from build123d import *

# Parameters (mm, degrees)
SKETCH1_W           = 300
SKETCH1_H           = 200
BOSS_EXTRUDE1_DEPTH = 60
FILLET1_R           = 5
SHELL1_START        = -145
SHELL1_OUTLINE_W    = 190
SHELL1_OUTLINE_H    = 115
SHELL1_DEPTH        = 290
SKETCH5_W           = 110
SKETCH5_H           = 180
CUT_EXTRUDE1_DEPTH  = 2.5
SKETCH6_W           = 110
SKETCH6_H           = 180
CUT_EXTRUDE2_DEPTH  = 2.5
SKETCH7_R           = 8.25
CUT_EXTRUDE3_DEPTH  = 320.540685985


# Read off the part's stored shape, not the designer's step: Shell1
with BuildPart() as part:
    # Sketch1 → Boss-Extrude1 (new, symmetric)
    with BuildSketch(Plane.XY):
        Rectangle(SKETCH1_W, SKETCH1_H)
    extrude(amount=BOSS_EXTRUDE1_DEPTH, both=True)

    # Fillet1
    fillet1_edges = [part.edges().sort_by_distance(p)[0] for p in [
        (150, -100, 0),
        (-150, -100, 0),
        (-150, 100, 0),
        (150, 100, 0),
    ]]
    fillet(fillet1_edges, radius=FILLET1_R)

    # Shell1 outline → Shell1 (cut)
    with BuildSketch(Plane.YZ.offset(SHELL1_START)):
        with Locations((0, 2.5)):
            Rectangle(SHELL1_OUTLINE_W, SHELL1_OUTLINE_H)
    extrude(amount=SHELL1_DEPTH, mode=Mode.SUBTRACT)

    # Sketch5 → Cut-Extrude1 (cut)
    with BuildSketch(Plane(origin=(150, 0, 0), x_dir=(0, 0, -1), z_dir=(1, 0, 0))):
        Rectangle(SKETCH5_W, SKETCH5_H)
    extrude(amount=-CUT_EXTRUDE1_DEPTH, mode=Mode.SUBTRACT)

    # Sketch6 → Cut-Extrude2 (cut)
    with BuildSketch(Plane.ZY.offset(150)):
        Rectangle(SKETCH6_W, SKETCH6_H)
    extrude(amount=-CUT_EXTRUDE2_DEPTH, mode=Mode.SUBTRACT)

    # Sketch7 → Cut-Extrude3 (cut, through all)
    with BuildSketch(Plane.ZY.offset(147.5)):
        with Locations((0, 43.15529971)):
            Circle(SKETCH7_R)
        with Locations((0, -26.84470029)):
            Circle(SKETCH7_R)
    extrude(amount=-CUT_EXTRUDE3_DEPTH, mode=Mode.SUBTRACT)


solid = part.part
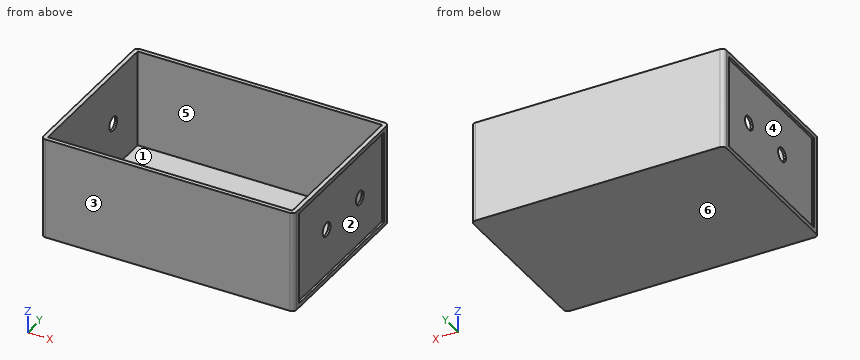
Could you check a few things on this model? Use its own coordinates, in mm. Face numbers are marked on the shaded views. A direction names the side the tool comes from. Coordinates: 2 decimals unless noted, no trailing zeros. Loops run counter-clockwise (first coordinate to the right, second up) from the corner with the lowest first, then second, coordinate; pieces in that order, holes last. Notation, with made-up numbers: (61, 9) -> (100, 9) arc R17 cw to (100, 39) -> close; hole circle Ø4 at (-29.75, -32.75). An arc over 180 degrees is marked (long way). Answer in a Markdown table with one row per item.
(1) For the marked faces 4, 5 and 6, which set-ups out of +Z, -Z, +X, -X, +Y, -Y let a thin tool reach every point of the face, with its end or its side?
Results found:
| item | result |
|---|---|
| face 4 | -X |
| face 5 | +Z |
| face 6 | -Z, +X, -X, +Y, -Y |
(2) Imagine slicing it at A-A (z = -49). List the corners of the cut face in (x, y) for me.
Results found:
| item | result |
|---|---|
| outline | (-150, -95) arc R5 ccw to (-145, -100) -> (145, -100) arc R5 ccw to (150, -95) -> (150, -90) -> (147.5, -90) -> (147.5, 90) -> (150, 90) -> (150, 95) arc R5 ccw to (145, 100) -> (-145, 100) arc R5 ccw to (-150, 95) -> (-150, 90) -> (-147.5, 90) -> (-147.5, -90) -> (-150, -90) -> close; hole (-145, -95) -> (145, -95) -> (145, 95) -> (-145, 95) -> close |
(3) Imagine slicing it at B-B (x = 99). List the corners of the cut face in (y, z) for me.
Results found:
| item | result |
|---|---|
| outline | (-100, -60) -> (100, -60) -> (100, 60) -> (95, 60) -> (95, -55) -> (-95, -55) -> (-95, 60) -> (-100, 60) -> close |
(4) Imagine slicing it at D-D (z = 0). Give the number of separate pieces and of enclosed holes in the cut face, plus the area to 3 significant figures.
Results found:
| item | result |
|---|---|
| separate pieces | 4 |
| enclosed holes | 0 |
| area | 3,810 mm^2 |
(5) Imagine slicing it at C-C (y = 71). List the corners of the cut face in (x, z) for me.
Results found:
| item | result |
|---|---|
| outline | (-150, -60) -> (150, -60) -> (150, -55) -> (147.5, -55) -> (147.5, 55) -> (150, 55) -> (150, 60) -> (145, 60) -> (145, -55) -> (-145, -55) -> (-145, 60) -> (-150, 60) -> (-150, 55) -> (-147.5, 55) -> (-147.5, -55) -> (-150, -55) -> close |
(6) If I drill on probe 1 along X at (y, z) = (8.5, -12.5); probe 2 along Y at (x, z) = (96, -53.5); probe 3 along Y at (x, z) = (-146, 0), over which ranges is the centre line in solid material (lowest first)?
Results found:
| item | result |
|---|---|
| probe 1 | x = -147.5 to -145, 145 to 147.5 |
| probe 2 | y = -100 to -95, 95 to 100 |
| probe 3 | y = -99.9 to -35.09, -18.59 to 34.91, 51.41 to 99.9 |
(7) Will these pins go through, and if not, where does the flat tip stop? pin 1 Ø10 at (y, z) = (10.5, -20) entering from +X; pin 2 Ø1.5 at (x, y) = (49, 68.5) entering from +Z; pin 3 Ø1.2 at (x, z) = (148.5, -18) entering from +Y.
Results found:
| item | result |
|---|---|
| pin 1 | stops at x = 147.5 |
| pin 2 | stops at z = -55 |
| pin 3 | stops at y = 99.07 |
(8) Thinking about a two-plate mould opening in X: for the marked faces 1, 2 and 3, which applies, released by +X, released by -X, zero draft, split by the parting line, or undercut?
Results found:
| item | result |
|---|---|
| face 1 | undercut |
| face 2 | released by +X |
| face 3 | zero draft |
